Verification items for the finished model (mm, model axes). A direction names the side the tool comes from. Coordinates: 2 decimals unless noted, no trailing zeros. Write each loop counter-clockwise with the first axis right and the second up, starting at its lowest first coordinate (ties: lowest second). Pieces come first, ordered by that corner, then holes. Notation, with made-up numbers: (62, 23) -> (75, 23) arc R16 cw to (75, 43) -> close; hole circle Ø5 at (-9.5, -10). An arc over 180 degrees is marked (long way). Write item = value, one per line. Start each with the question number.
(1) Section check B-B (z = 27.5). Record the cut outline in (x, y) (3 decimals), plus the area to 3 significant figures.
(2) Section check C-C (y = 11.43). Record the cut outline in (x, z) (1 decimal).
(3) Mould release check, pull along Y, two halves, no side actions. Record for faces 4 (the face through (-1, 30.48, 16)), 5 (the face through (52, 20.904, 16)), 6 (the face through (-1, -30.48, 16)): released by +Y, released by -Y, zero draft, split by the parting line, or undercut.
(4) Section check D-D (z = 10.16). State how many separate pieces and enclosed holes the cut face has, plus the area to 3 significant figures.
(5) Material ranges on probe 1 along X at (y, z) = (23.5, 10); probe 2 along X at (y, z) = (25.5, 16); probe 3 along X at (y, z) = (7.5, 4.5), recorded low to high. Write a range as [from, to].
(6) Set-up check for faces 1 (the face through (-55, -29.5, 16.2)), 2 (the face through (54.916, -5.856, 12.315)), 3 (the face through (-1, -28.524, 16)): record each of +Z, -Z, +X, -X, +Y, -Y from which the full face is reachable in a straight line by a thin tool's end or side.
(7) Gauge pin test, flat ends, axial feed: pin 1 Ø4 at (x, y) = (-39, 14) entering from +Z; pin 2 Ø2.5 at (x, y) = (-51, -25) entering from +Z. Record the tip position at first contact, or that the pin passes through.
(8) Section check A-A (y = 0). Record the cut outline in (x, z) (1 decimal).
```python
from build123d import *

# Parameters (mm, degrees)
F0_W      = 111.76
F0_H      = 60.96
F1_DEPTH  = 30.48
F2_T      = -1.9558
F4_DEPTH  = 28.5242
F5_R      = 2.54
F6_DEPTH  = 25.4
F9_R      = 3.175
F10_R     = 1.5875
F11_R     = 7.1755
F12_DEPTH = 1.9558
F13_R     = 6.0325
F14_DEPTH = 1.9558
F15_R     = 9.525
F16_DEPTH = 30.481


with BuildPart() as f1:
    # F0 (on Top) → F1 (new body)
    with BuildSketch(Plane.XY):
        Rectangle(F0_W, F0_H)
    extrude(amount=F1_DEPTH)

    # F2
    f2_openings = [f1.faces().sort_by_distance(p)[0] for p in [
        (0, 0, 30.48),
    ]]
    offset(amount=F2_T, openings=f2_openings)

    # F3 (on face) → F4 (join, through all)
    with BuildSketch(Plane.XY.offset(30.48)):
        with BuildLine():
            Line((-53.9242, 20.9042), (-50.1142, 20.9042))
            ThreePointArc((-50.1142, 20.9042), (-47.4201231637, 22.0201231637), (-46.3042, 24.7142))
            Line((-46.3042, 24.7142), (-46.3042, 28.5242))
            Line((-46.3042, 28.5242), (-53.9242, 28.5242))
            Line((-53.9242, 28.5242), (-53.9242, 20.9042))
        make_face()
    extrude(amount=-F4_DEPTH)

    # F5 (on face) → F6 (cut)
    with BuildSketch(Plane.XY.offset(30.48)):
        with Locations((-50.1142, 24.7142)):
            Circle(F5_R)
    extrude(amount=-F6_DEPTH, mode=Mode.SUBTRACT)

    # F7: F1 across plane


with BuildPart() as f1_1:
    add(f1.part)
    add(f1.part.mirror(Plane.YZ))

    # F8: F1 across plane


with BuildPart() as f1_2:
    add(f1_1.part)
    add(f1_1.part.mirror(Plane.XZ))

    # F9
    f9_edges = [f1_2.edges().sort_by_distance(p)[0] for p in [
        (-55.88, 30.48, 15.24),
        (-55.88, -30.48, 15.24),
        (55.88, -30.48, 15.24),
        (55.88, 30.48, 15.24),
    ]]
    fillet(f9_edges, radius=F9_R)

    # F10
    f10_edges = [f1_2.edges().sort_by_distance(p)[0] for p in [
        (0, -30.48, 0),
        (-54.950064, -29.550064, 0),
        (54.950064, -29.550064, 0),
        (-55.88, 0, 0),
        (55.88, 0, 0),
        (-54.950064, 29.550064, 0),
        (54.950064, 29.550064, 0),
        (0, 30.48, 0),
    ]]
    fillet(f10_edges, radius=F10_R)

    # F11 (on face) → F12 (cut, through all)
    with BuildSketch(Plane.YZ.offset(55.88)):
        with Locations((-12.7, 10.16)):
            Circle(F11_R)
    extrude(amount=-F12_DEPTH, mode=Mode.SUBTRACT)

    # F13 (on face) → F14 (cut, through all)
    with BuildSketch(Plane.YZ.offset(55.88)):
        with Locations((11.43, 17.78)):
            Circle(F13_R)
    extrude(amount=-F14_DEPTH, mode=Mode.SUBTRACT)

    # F15 (on face) → F16 (cut, through all)
    with BuildSketch(Plane(origin=(0, 0, 0), x_dir=(1, 0, 0), z_dir=(0, 0, -1))):
        with Locations((-25.4, 0)):
            Circle(F15_R)
    extrude(amount=-F16_DEPTH, mode=Mode.SUBTRACT)


solid = f1_2.part
```
Response:
q1.outline = (-55.88, -27.305) arc R3.175 ccw to (-52.705, -30.48) -> (52.705, -30.48) arc R3.175 ccw to (55.88, -27.305) -> (55.88, 27.305) arc R3.175 ccw to (52.705, 30.48) -> (-52.705, 30.48) arc R3.175 ccw to (-55.88, 27.305) -> close; hole (-53.924, -20.904) -> (-50.114, -20.904) arc R3.81 cw to (-46.304, -24.714) -> (-46.304, -28.524) -> (46.304, -28.524) -> (46.304, -24.714) arc R3.81 cw to (50.114, -20.904) -> (53.924, -20.904) -> (53.924, 20.904) -> (50.114, 20.904) arc R3.81 cw to (46.304, 24.714) -> (46.304, 28.524) -> (-46.304, 28.524) -> (-46.304, 24.714) arc R3.81 cw to (-50.114, 20.904) -> (-53.924, 20.904) -> close; hole circle Ø5.08 at (-50.114, -24.714); hole circle Ø5.08 at (-50.114, 24.714); hole circle Ø5.08 at (50.114, -24.714); hole circle Ø5.08 at (50.114, 24.714)
q1.area = 790 mm2
q2.outline = (-55.9, 1.6) arc R1.6 ccw to (-54.3, 0) -> (54.3, 0) arc R1.6 ccw to (55.9, 1.6) -> (55.9, 11.7) -> (53.9, 11.7) -> (53.9, 2) -> (-53.9, 2) -> (-53.9, 30.5) -> (-55.9, 30.5) -> close; (53.9, 23.8) -> (55.9, 23.8) -> (55.9, 30.5) -> (53.9, 30.5) -> close
q3.face_4 = released by +Y
q3.face_5 = undercut
q3.face_6 = released by -Y
q4.separate_pieces = 1
q4.enclosed_holes = 4
q4.area = 762 mm2
q5.probe_1 = [-55.88, -52.35], [-47.88, -46.5], [46.5, 47.88], [52.35, 55.88]
q5.probe_2 = [-55.88, -52.53], [-47.7, -46.3], [46.3, 47.7], [52.53, 55.88]
q5.probe_3 = [-55.88, -53.92], [53.92, 55.88]
q6.face_1 = +Z, -Z, -X, -Y
q6.face_2 = +X
q6.face_3 = +Z
q7.pin_1 = 1.96
q7.pin_2 = 5.08
q8.outline = (-55.9, 1.6) arc R1.6 ccw to (-54.3, 0) -> (-34.9, 0) -> (-34.9, 2) -> (-53.9, 2) -> (-53.9, 30.5) -> (-55.9, 30.5) -> close; (-15.9, 0) -> (54.3, 0) arc R1.6 ccw to (55.9, 1.6) -> (55.9, 30.5) -> (53.9, 30.5) -> (53.9, 2) -> (-15.9, 2) -> close
